```python
from build123d import *

# Parameters (mm, degrees)
STOCK_D_1_OUTLINE_W     = 100
STOCK_D_1_OUTLINE_H     = 100
STOCK_D_1_DEPTH         = 3
STOCK_D_1_START         = 3
STOCK_D_1_2_OUTLINE_W   = 100
STOCK_D_1_2_OUTLINE_H   = 100
STOCK_D_1_2_OUTLINE_W_2 = 94
STOCK_D_1_2_OUTLINE_H_2 = 94
STOCK_D_1_2_DEPTH       = 14.5
SKETCH1_W               = 10
SKETCH1_H               = 10
BOSS_EXTRUDE1_DEPTH     = 5
CUT_EXTRUDE1_DEPTH      = 143.162758836
CUT_EXTRUDE1_DEPTH_BACK = 143.162758836
SKETCH3_R               = 1.35
SKETCH22_W              = 3
SKETCH22_H              = 10
BOSS_EXTRUDE7_DEPTH     = 5
FILLET8_R               = 4
BOSS_EXTRUDE5_DEPTH     = 2.5
SKETCH14_R              = 3.5
BOSS_EXTRUDE6_DEPTH     = 2.5
CUT_EXTRUDE2_REACH      = 144.5
SKETCH5_W               = 62.5
SKETCH5_H               = 6
SKETCH11_W              = 62.5
SKETCH11_H              = 6
BOSS_EXTRUDE3_DEPTH     = 8.5
SKETCH13_W              = 5.75
SKETCH13_H              = 6
BOSS_EXTRUDE4_DEPTH     = 14.5
SKETCH16_R              = 1.35
CUT_EXTRUDE3_DEPTH      = 8
CUT_EXTRUDE4_REACH      = 144.5
SKETCH17_W              = 43
SKETCH17_H              = 4.5
CUT_EXTRUDE5_REACH      = 144.5
SKETCH18_W              = 56
SKETCH18_H              = 8.5
FILLET10_R              = 2
FILLET11_R              = 2
FILLET13_R              = 1.5
FILLET14_R              = 4
CUT_EXTRUDE7_REACH      = 144.163
SKETCH23_W              = 12
SKETCH23_H              = 12
BOSS_EXTRUDE8_DEPTH     = 5
SKETCH24_R              = 2.65
CUT_EXTRUDE8_DEPTH      = 151.666021385
SKETCH26_W              = 5
SKETCH26_H              = 12
BOSS_EXTRUDE9_DEPTH     = 17.5
CHAMFER3_SIZE           = 12


with BuildPart() as part:
    # Stock-Dėžė-1: read off the stored shape, not the designer's step
    # Stock-Dėžė-1 outline → Stock-Dėžė-1 (new body)
    with BuildSketch(Plane(origin=(0, 0, 0), x_dir=(1, 0, 0), z_dir=(0, 1, 0))):
        with Locations((50, -50)):
            Rectangle(STOCK_D_1_OUTLINE_W, STOCK_D_1_OUTLINE_H)
    extrude(amount=STOCK_D_1_DEPTH)

    # Stock-D_-1 2 outline → Stock-D_-1 2 (add)
    with BuildSketch(Plane(origin=(0, 0, 0), x_dir=(1, 0, 0), z_dir=(0, 1, 0)).offset(STOCK_D_1_START)):
        with Locations((50, -50)):
            Rectangle(STOCK_D_1_2_OUTLINE_W, STOCK_D_1_2_OUTLINE_H)
        with Locations((50, -50)):
            Rectangle(STOCK_D_1_2_OUTLINE_W_2, STOCK_D_1_2_OUTLINE_H_2, mode=Mode.SUBTRACT)
    extrude(amount=STOCK_D_1_2_DEPTH)

    # Sketch1 → Boss-Extrude1 (add)
    with BuildSketch(Plane(origin=(0, 3, 0), x_dir=(1, 0, 0), z_dir=(0, 1, 0))):
        with Locations((8, -8)):
            Rectangle(SKETCH1_W, SKETCH1_H)
        with Locations((92, -8)):
            Rectangle(SKETCH1_W, SKETCH1_H)
        with Locations((11, -92)):
            Rectangle(SKETCH1_W, SKETCH1_H)
    extrude(amount=BOSS_EXTRUDE1_DEPTH)

    # Sketch3 → Cut-Extrude1 (cut, two sides: drawn at the far end of the back side and taken through both)
    with BuildSketch(Plane(origin=(0, 3, 0), x_dir=(1, 0, 0), z_dir=(0, 1, 0)).offset(-CUT_EXTRUDE1_DEPTH_BACK)):
        with Locations(Location((8, -8, 0), (0, 0, 270))):
            Circle(SKETCH3_R)
        with Locations(Location((11, -92, 0), (0, 0, 90))):
            Circle(SKETCH3_R)
        with Locations(Location((92, -8, 0), (0, 0, 90))):
            Circle(SKETCH3_R)
    extrude(amount=CUT_EXTRUDE1_DEPTH + CUT_EXTRUDE1_DEPTH_BACK, mode=Mode.SUBTRACT)

    # Sketch22 → Boss-Extrude7 (add)
    with BuildSketch(Plane(origin=(0, 3, 0), x_dir=(1, 0, 0), z_dir=(0, 1, 0))):
        with Locations((4.5, -92)):
            Rectangle(SKETCH22_W, SKETCH22_H)
    extrude(amount=BOSS_EXTRUDE7_DEPTH)

    # Fillet8
    fillet8_edges = [part.edges().sort_by_distance(p)[0] for p in [
        (3, 5.5, 13),
        (13, 5.5, 13),
        (97, 5.5, 13),
        (87, 5.5, 13),
        (16, 5.5, 97),
        (16, 5.5, 87),
        (3, 5.5, 87),
    ]]
    fillet(fillet8_edges, radius=FILLET8_R)

    # Sketch6 → Boss-Extrude5 (add)
    with BuildSketch(Plane(origin=(0, 3, 0), x_dir=(1, 0, 0), z_dir=(0, 1, 0))):
        with BuildLine():
            Line((64, -92), (64, -97))
            Line((64, -97), (74, -97))
            Line((74, -97), (74, -92))
            Line((74, -92), (74, -43))
            ThreePointArc((74, -43), (72.535533906, -39.464466094), (69, -38))
            Line((69, -38), (8, -38))
            Line((8, -38), (3, -38))
            Line((3, -38), (3, -48))
            Line((3, -48), (64, -48))
            Line((64, -48), (64, -92))
        make_face()
    extrude(amount=BOSS_EXTRUDE5_DEPTH)

    # Sketch14 → Boss-Extrude6 (add)
    with BuildSketch(Plane(origin=(0, 5.5, 0), x_dir=(1, 0, 0), z_dir=(0, 1, 0))):
        with Locations(Location((69, -43, 0), (0, 0, 270))):
            Circle(SKETCH14_R)
        with BuildLine():
            Line((11, -40), (3, -40))
            Line((3, -40), (3, -46))
            Line((3, -46), (11, -46))
            ThreePointArc((11, -46), (14, -43), (11, -40))
        make_face()
        with BuildLine():
            Line((72, -92), (72, -97))
            Line((72, -97), (66, -97))
            Line((66, -97), (66, -92))
            ThreePointArc((66, -92), (69, -89), (72, -92))
        make_face()
    extrude(amount=BOSS_EXTRUDE6_DEPTH)

    # Sketch5 → Cut-Extrude2 (cut, up to next)
    with BuildSketch(Plane(origin=(0, 0, 0), x_dir=(-1, 0, 0), z_dir=(0, 0, -1)), mode=Mode.PRIVATE) as cut_extrude2_sk1:
        with Locations((-50, 14.5)):
            Rectangle(SKETCH5_W, SKETCH5_H)
    cut_extrude2_tool1 = extrude(cut_extrude2_sk1.sketch, amount=-CUT_EXTRUDE2_REACH, mode=Mode.PRIVATE) & part.part
    add(cut_extrude2_tool1.solids().sort_by_distance((50, 14.5, 0))[0], mode=Mode.SUBTRACT)

    # Sketch11 → Boss-Extrude3 (add)
    with BuildSketch(Plane(origin=(0, 3, 0), x_dir=(1, 0, 0), z_dir=(0, 1, 0))):
        with Locations((50, -6)):
            Rectangle(SKETCH11_W, SKETCH11_H)
    extrude(amount=BOSS_EXTRUDE3_DEPTH)

    # Sketch13 → Boss-Extrude4 (add)
    with BuildSketch(Plane(origin=(0, 3, 0), x_dir=(1, 0, 0), z_dir=(0, 1, 0))):
        with Locations((15.875, -6)):
            Rectangle(SKETCH13_W, SKETCH13_H)
        with Locations((84.125, -6)):
            Rectangle(SKETCH13_W, SKETCH13_H)
    extrude(amount=BOSS_EXTRUDE4_DEPTH)

    # Sketch16 → Cut-Extrude3 (cut)
    with BuildSketch(Plane(origin=(0, 8, 0), x_dir=(1, 0, 0), z_dir=(0, 1, 0))):
        with Locations(Location((69, -43, 0), (0, 0, 270))):
            Circle(SKETCH16_R)
        with Locations(Location((11, -43, 0), (0, 0, 270))):
            Circle(SKETCH16_R)
        with Locations(Location((69, -92, 0), (0, 0, 270))):
            Circle(SKETCH16_R)
    extrude(amount=-CUT_EXTRUDE3_DEPTH, mode=Mode.SUBTRACT)

    # Sketch17 → Cut-Extrude4 (cut, up to next)
    with BuildSketch(Plane.XY.offset(100), mode=Mode.PRIVATE) as cut_extrude4_sk1:
        with Locations((32.5, 11.45)):
            Rectangle(SKETCH17_W, SKETCH17_H)
    cut_extrude4_tool1 = extrude(cut_extrude4_sk1.sketch, amount=-CUT_EXTRUDE4_REACH, mode=Mode.PRIVATE) & part.part
    add(cut_extrude4_tool1.solids().sort_by_distance((32.5, 11.45, 100))[0], mode=Mode.SUBTRACT)

    # Sketch18 → Cut-Extrude5 (cut, up to next)
    with BuildSketch(Plane(origin=(100, 0, 0), x_dir=(0, 0, -1), z_dir=(1, 0, 0)), mode=Mode.PRIVATE) as cut_extrude5_sk1:
        with Locations((-66, 13.25)):
            Rectangle(SKETCH18_W, SKETCH18_H)
    cut_extrude5_tool1 = extrude(cut_extrude5_sk1.sketch, amount=-CUT_EXTRUDE5_REACH, mode=Mode.PRIVATE) & part.part
    add(cut_extrude5_tool1.solids().sort_by_distance((100, 13.25, 66))[0], mode=Mode.SUBTRACT)

    # Fillet10
    fillet10_edges = [part.edges().sort_by_distance(p)[0] for p in [
        (87, 5.5, 9),
        (13, 5.5, 9),
    ]]
    fillet(fillet10_edges, radius=FILLET10_R)

    # Fillet11
    fillet11_edges = [part.edges().sort_by_distance(p)[0] for p in [
        (64, 4.25, 48),
        (64, 4.25, 97),
        (74, 4.25, 97),
        (3, 4.25, 38),
        (3, 4.25, 48),
    ]]
    fillet(fillet11_edges, radius=FILLET11_R)

    # Fillet13
    fillet13_edges = [part.edges().sort_by_distance(p)[0] for p in [
        (13, 12.75, 9),
        (87, 12.75, 9),
    ]]
    fillet(fillet13_edges, radius=FILLET13_R)

    # Fillet14
    fillet14_edges = [part.edges().sort_by_distance(p)[0] for p in [
        (72, 6.75, 97),
        (66, 6.75, 97),
        (3, 6.75, 40),
        (3, 6.75, 46),
    ]]
    fillet(fillet14_edges, radius=FILLET14_R)

    # Sketch21 → Cut-Extrude7 (cut, up to next)
    with BuildSketch(Plane(origin=(0, 3, 0), x_dir=(1, 0, 0), z_dir=(0, 1, 0)), mode=Mode.PRIVATE) as cut_extrude7_sk1:
        with BuildLine():
            Line((60, -52.5), (60, -92.5))
            ThreePointArc((60, -92.5), (57.8, -94.7), (55.6, -92.5))
            Line((55.6, -92.5), (55.6, -52.5))
            ThreePointArc((55.6, -52.5), (57.8, -50.3), (60, -52.5))
        make_face()
    cut_extrude7_tool1 = extrude(cut_extrude7_sk1.sketch, amount=-CUT_EXTRUDE7_REACH, mode=Mode.PRIVATE) & part.part
    # Sketch21 → Cut-Extrude7 (cut, up to next)
    with BuildSketch(Plane(origin=(0, 3, 0), x_dir=(1, 0, 0), z_dir=(0, 1, 0)), mode=Mode.PRIVATE) as cut_extrude7_sk2:
        with BuildLine():
            Line((46.1, -52.5), (46.1, -92.5))
            ThreePointArc((46.1, -92.5), (48.3, -94.7), (50.5, -92.5))
            Line((50.5, -92.5), (50.5, -52.5))
            ThreePointArc((50.5, -52.5), (48.3, -50.3), (46.1, -52.5))
        make_face()
    cut_extrude7_tool2 = extrude(cut_extrude7_sk2.sketch, amount=-CUT_EXTRUDE7_REACH, mode=Mode.PRIVATE) & part.part
    # Sketch21 → Cut-Extrude7 (cut, up to next)
    with BuildSketch(Plane(origin=(0, 3, 0), x_dir=(1, 0, 0), z_dir=(0, 1, 0)), mode=Mode.PRIVATE) as cut_extrude7_sk3:
        with BuildLine():
            Line((36.6, -52.5), (36.6, -92.5))
            ThreePointArc((36.6, -92.5), (38.8, -94.7), (41, -92.5))
            Line((41, -92.5), (41, -52.5))
            ThreePointArc((41, -52.5), (38.8, -50.3), (36.6, -52.5))
        make_face()
    cut_extrude7_tool3 = extrude(cut_extrude7_sk3.sketch, amount=-CUT_EXTRUDE7_REACH, mode=Mode.PRIVATE) & part.part
    # Sketch21 → Cut-Extrude7 (cut, up to next)
    with BuildSketch(Plane(origin=(0, 3, 0), x_dir=(1, 0, 0), z_dir=(0, 1, 0)), mode=Mode.PRIVATE) as cut_extrude7_sk4:
        with BuildLine():
            Line((27.1, -52.5), (27.1, -92.5))
            ThreePointArc((27.1, -92.5), (29.3, -94.7), (31.5, -92.5))
            Line((31.5, -92.5), (31.5, -52.5))
            ThreePointArc((31.5, -52.5), (29.3, -50.3), (27.1, -52.5))
        make_face()
    cut_extrude7_tool4 = extrude(cut_extrude7_sk4.sketch, amount=-CUT_EXTRUDE7_REACH, mode=Mode.PRIVATE) & part.part
    # Sketch21 → Cut-Extrude7 (cut, up to next)
    with BuildSketch(Plane(origin=(0, 3, 0), x_dir=(1, 0, 0), z_dir=(0, 1, 0)), mode=Mode.PRIVATE) as cut_extrude7_sk5:
        with BuildLine():
            Line((17.6, -52.5), (17.6, -92.5))
            ThreePointArc((17.6, -92.5), (19.8, -94.7), (22, -92.5))
            Line((22, -92.5), (22, -52.5))
            ThreePointArc((22, -52.5), (19.8, -50.3), (17.6, -52.5))
        make_face()
    cut_extrude7_tool5 = extrude(cut_extrude7_sk5.sketch, amount=-CUT_EXTRUDE7_REACH, mode=Mode.PRIVATE) & part.part
    # Sketch21 → Cut-Extrude7 (cut, up to next)
    with BuildSketch(Plane(origin=(0, 3, 0), x_dir=(1, 0, 0), z_dir=(0, 1, 0)), mode=Mode.PRIVATE) as cut_extrude7_sk6:
        with BuildLine():
            Line((7.3, -52.5), (7.3, -82.5))
            ThreePointArc((7.3, -82.5), (9.5, -84.7), (11.7, -82.5))
            Line((11.7, -82.5), (11.7, -52.5))
            ThreePointArc((11.7, -52.5), (9.5, -50.3), (7.3, -52.5))
        make_face()
    cut_extrude7_tool6 = extrude(cut_extrude7_sk6.sketch, amount=-CUT_EXTRUDE7_REACH, mode=Mode.PRIVATE) & part.part
    add(cut_extrude7_tool1.solids().sort_by_distance((57.8, 3, 72.5))[0], mode=Mode.SUBTRACT)
    add(cut_extrude7_tool2.solids().sort_by_distance((48.3, 3, 72.5))[0], mode=Mode.SUBTRACT)
    add(cut_extrude7_tool3.solids().sort_by_distance((38.8, 3, 72.5))[0], mode=Mode.SUBTRACT)
    add(cut_extrude7_tool4.solids().sort_by_distance((29.3, 3, 72.5))[0], mode=Mode.SUBTRACT)
    add(cut_extrude7_tool5.solids().sort_by_distance((19.8, 3, 72.5))[0], mode=Mode.SUBTRACT)
    add(cut_extrude7_tool6.solids().sort_by_distance((9.5, 3, 67.5))[0], mode=Mode.SUBTRACT)

    # Sketch23 → Boss-Extrude8 (add)
    with BuildSketch(Plane.XZ):
        with Locations((11, 106)):
            Rectangle(SKETCH23_W, SKETCH23_H)
        with Locations((89, 106)):
            Rectangle(SKETCH23_W, SKETCH23_H)
    extrude(amount=-BOSS_EXTRUDE8_DEPTH)

    # Sketch24 → Cut-Extrude8 (cut, through all)
    with BuildSketch(Plane(origin=(0, 5, 0), x_dir=(1, 0, 0), z_dir=(0, 1, 0))):
        with Locations(Location((11, -106, 0), (0, 0, 270))):
            Circle(SKETCH24_R)
        with Locations(Location((89, -106, 0), (0, 0, 270))):
            Circle(SKETCH24_R)
    extrude(amount=-CUT_EXTRUDE8_DEPTH, mode=Mode.SUBTRACT)

    # Sketch26 → Boss-Extrude9 (add)
    with BuildSketch(Plane.XZ):
        with Locations((2.5, 106)):
            Rectangle(SKETCH26_W, SKETCH26_H)
        with Locations((97.5, 106)):
            Rectangle(SKETCH26_W, SKETCH26_H)
    extrude(amount=-BOSS_EXTRUDE9_DEPTH)

    # Chamfer3
    chamfer3_edges = [part.edges().sort_by_distance(p)[0] for p in [
        (17, 2.5, 100),
        (83, 2.5, 100),
    ]]
    chamfer(chamfer3_edges, length=CHAMFER3_SIZE - 0.0001)  # a hair under: the kernel refuses the full size


solid = part.part
```
Part model, mm, in its own coordinate system. A direction names the side the tool comes from. Round coordinates to 2 decimals unless told otherwise and drop trailing zeros. Loops run counter-clockwise (first coordinate to the right, second up) from the corner with the lowest first, then second, coordinate; pieces in that order, holes last.
1. Slice it at A-A (x = 57.8). Give the cut face in (y, z).
Solutions:
outline: (0, 0) - (11.5, 0) - (11.5, 9) - (3, 9) - (3, 38) - (5.5, 38) - (5.5, 48) - (3, 48) - (3, 50.3) - (0, 50.3) - close; (0, 94.7) - (3, 94.7) - (3, 97) - (17.5, 97) - (17.5, 100) - (0, 100) - close
2. Slice it at B-B (x = 38.8). Give the cut face in (y, z).
Solutions:
outline: (0, 0) - (11.5, 0) - (11.5, 9) - (3, 9) - (3, 38) - (5.5, 38) - (5.5, 48) - (3, 48) - (3, 50.3) - (0, 50.3) - close; (0, 94.7) - (3, 94.7) - (3, 97) - (9.2, 97) - (9.2, 100) - (0, 100) - close; (13.7, 97) - (17.5, 97) - (17.5, 100) - (13.7, 100) - close
3. Slice it at D-D (y = 1.25). Count the separate pieces of the cut face and the enclosed holes in it, and give its area (3 significant figures).
Solutions:
separate pieces: 1
enclosed holes: 14
area: 9,370 mm2
4. Two-plate mould, pull along X, no slides. Class faces 1 (the face through (0, 9, 55)), 2 (the face through (74, 4, 69)), 3 (the face through (100, 7, 57)): pulls with the +X half, pulls with the -X half, needs draft (parallel to the pull), parting line crosses it, or undercut.
Solutions:
face 1: pulls with the -X half
face 2: undercut
face 3: pulls with the +X half
5. Flat gauge pins, fed straight in: pin 1 (5.5 mm diameter, centred on x = 67.5, z = 41.5, fed in from +Y); pin 2 (1.2 mm diameter, centred on x = 9.5, y = 7, fed in from +Z); pin 3 (9.5 mm diameter, centred on x = 85, z = 106, fed in from +Y); pin 4 (3 mm diameter, centred on x = 89, z = 106, fed in from +Y). Where does each tip first touch, or does it go through?
Solutions:
pin 1: stops at y = 8
pin 2: stops at z = 100
pin 3: stops at y = 5
pin 4: passes through
6. 3-axis set-ups, long thin cutter, end or side, ignore diameter. For faces 4 (the face through (33, 3, 72)), 5 (the face through (29.3, 1.5, 94.7)), 6 (the face through (18.75, 14, 5)), 7 (the face through (14, 5, 105)): which of +Z, -Z, +X, -X, +Y, -Y reach the whole face in a straight line?
Solutions:
face 4: +Y
face 5: +Y, -Y
face 6: -Z, +Y
face 7: +Z, +Y
7. Slice it at C-C (z = 25). Give the cut face in (x, y).
Solutions:
outline: (0, 0) - (100, 0) - (100, 17.5) - (97, 17.5) - (97, 3) - (3, 3) - (3, 17.5) - (0, 17.5) - close
8. Drill centre lines: line 1 along Z through (x, y) = (8, 4); line 2 along X through (y, z) = (1.75, 90.5); line 3 along Z through (x, y) = (8, 2.75). Where is each one in solid material? Low to high.
Solutions:
line 1: z = 0 to 6.65, 9.35 to 13, 38 to 48, 87 to 112
line 2: x = 0 to 17.6, 22 to 27.1, 31.5 to 36.6, 41 to 46.1, 50.5 to 55.6, 60 to 100
line 3: z = 0 to 6.65, 9.35 to 50.89, 84.11 to 112
